Answer from the drawing. Dimensions are ordinates in mm from the lowest x, y and z of the part. A direction names the side the tool comes from. Coordinates: 2 decimals unless noted, no trailing zeros. Loops run counter-clockwise (first coordinate to the right, second up) from the corner with the lowest first, then second, coordinate; pieces in that order, holes last.
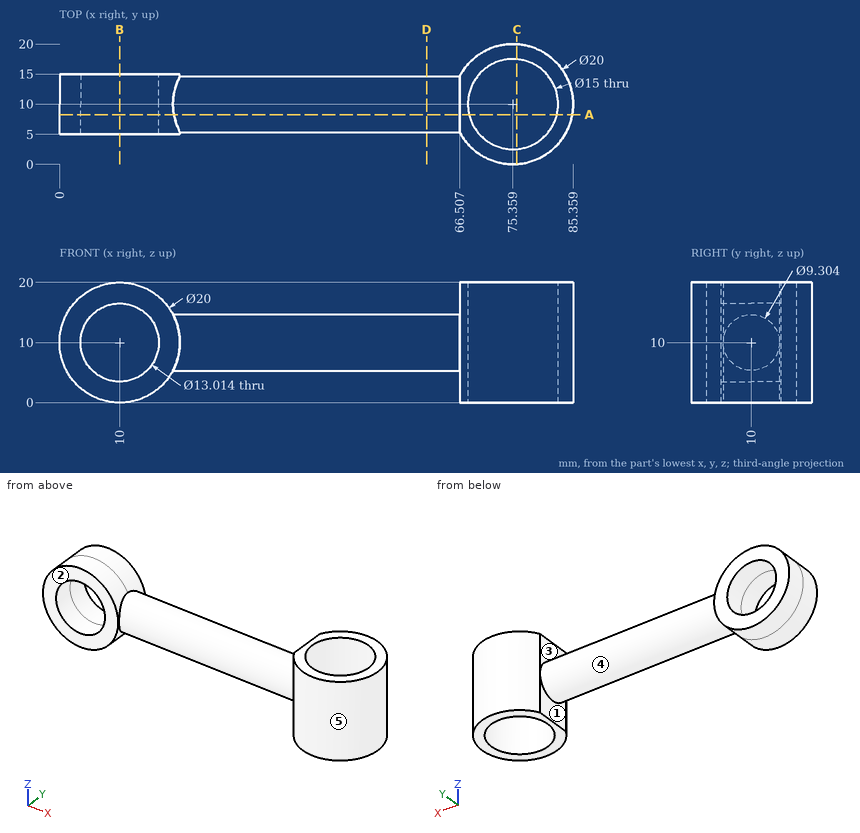
Item 1: A cutting plane is placed at B-B on x = 10. Determine the outline of the cut face in (y, z).
Numbers:
outline: (5, 0) - (15, 0) - (15, 3.49) - (5, 3.49) - close; (5, 16.51) - (15, 16.51) - (15, 20) - (5, 20) - close
Item 2: A cutting plane is placed at D-D on x = 61. Determine the outline of the cut face in (y, z).
Numbers:
outline: circle Ø9.3 at (10, 10)
Item 3: A cutting plane is placed at A-A on y = 8.25. Determine the outline of the cut face in (x, z) (1 decimal), then the cut area to 3 significant figures.
Numbers:
outline: (19, 5.7) - (66.5, 5.7) - (66.5, 0) - (68.1, 0) - (68.1, 20) - (66.5, 20) - (66.5, 14.3) - (19, 14.3) arc R10 ccw (long way) to start; (82.7, 0) - (85.2, 0) - (85.2, 20) - (82.7, 20) - close; hole circle Ø13 at (10, 10)
area: 667 mm2
Item 4: Given pin 1 (6 mm diameter, centred on x = 10.5, z = 11, fed in from -Y); pin 2 (1 mm diameter, centred on x = 68, z = 4.5, fed in from +Y); pin 3 (8 mm diameter, centred on x = 60, y = 9.5, fed in from -Z); pin 4 (6 mm diameter, centred on y = 9, z = 6.5, fed in from -X), each flat-ended and moving along its own axis, determine where each tip first touches the part or whether it passes through.
Numbers:
pin 1: passes through
pin 2: stops at y = 17.28
pin 3: stops at z = 5.35
pin 4: stops at x = 0.01
Item 5: Determine the mould class of the marked faces 1, 2 and 3 for opening direction X: released by +X, released by -X, zero draft, split by the parting line, or undercut.
Numbers:
face 1: undercut
face 2: zero draft
face 3: undercut
Item 6: A cutting plane is placed at C-C on x = 76. Determine the outline of the cut face in (y, z), then the cut area to 3 significant figures.
Numbers:
outline: (0.02, 0) - (2.53, 0) - (2.53, 20) - (0.02, 20) - close; (17.47, 0) - (19.98, 0) - (19.98, 20) - (17.47, 20) - close
area: 100 mm2
Item 7: Which of the six approach directions +Z, -Z, +X, -X, +Y, -Y give full straight-line access (tool end or side, diameter ignored) to the marked faces 4 and 5?
Numbers:
face 4: none
face 5: +Z, -Z
Item 8: Find the intervals of material crossed by line 1 along Z through (x, y) = (10, 8.5); line 2 along Z through (x, y) = (38.5, 10.25) (1 decimal); line 3 along X through (y, z) = (7.5, 17.5) (1 decimal), in increasing order.
Numbers:
line 1: z = 0 to 3.49, 16.51 to 20
line 2: z = 5.4 to 14.6
line 3: x = 3.4 to 16.6, 66.5 to 68.3, 82.4 to 85
